Design review of the part built by this model. Coordinates are the model's own, in mm. Face numbers are marked on the shaded views. Coordinates: 2 decimals unless noted, no trailing zeros. Loops run counter-clockwise (first coordinate to the right, second up) from the corner with the lowest first, then second, coordinate; pieces in that order, holes last.
Q1. Add section B-B on x = 13. Give the boundary of the cut face in (y, z).
Q2. Add section D-D on x = -5. Give the boundary of the cut face in (y, z).
Q3. Add section C-C on z = 0. Give the boundary of the cut face in (x, y), and give its area (3 significant figures).
Q4. Wall thickness on probe 1 along Z at (x, y) = (0, -1.5); probe 2 along X at (y, z) = (-1.5, 22.5); probe 3 along Z at (x, y) = (3, -0.5): over which ranges is each line inside the solid? List them lowest first.
Q5. Draft analysis for pull direction X (two halves, no side actions). For the marked faces 1, 2 and 3, state which applies: released by +X, released by -X, zero draft, split by the parting line, or undercut.
Q6. Add section A-A on x = 0. Give the boundary of the cut face in (y, z).
Q7. For P1, Ø2, axis at x = -11.5, y = 1, coming from the +Z side; P2, Ø1, axis at x = -3.5, y = -1, coming from the -Z side; P3, Ø3.5, axis at x = -2.5, z = 23, coming from the -Y side; P4, Ø5, axis at x = 0, z = -21.5, coming from the +Y side, all flat-tipped, find the tip position at first contact; note any pin that passes through.
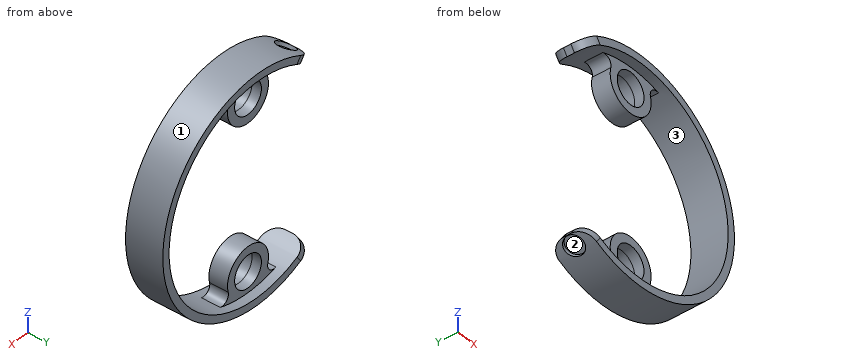
Autodesk Inventor part; units mm, degrees
ref_plane "YZ Plane" through (0, 0, 0) normal (1, 0, 0) x (0, 1, 0)
ref_plane "XZ Plane" through (0, 0, 0) normal (0, 1, 0) x (-1, 0, 0)
ref_plane "XY Plane" through (0, 0, 0) normal (0, 0, 1) x (1, 0, 0)
sketch "Skizze1" plane through (0, 0, 0) normal (0, 1, 0) x (-1, 0, 0)
  circle A0 centre (0, 0) radius 28
  circle A1 centre (0, 0) radius 30
  dimension "d0" = 56
  dimension "d1" = 60
extrude "Extrusion1" add sketch "Skizze1" along normal mid plane 10
sketch "Skizze2" plane through (0, 0, 0) normal (0, 1, 0) x (-1, 0, 0)
  circle A0 centre (0, 22.5) radius 4.25
  circle A1 centre (0, -22.5) radius 4.25
  line L0 (44.9262, 0) -> (-43.1306, 0) construction
  circle A2 centre (0, -22.5) radius 6.5
  circle A3 centre (0, 22.5) radius 6.5
  line L1 (0, 38.6377) -> (0, -60.2779) construction
  line L2 (3, 29.5) -> (-3, 29.5)
  line L3 (-3, 29.5) -> (-3, -29.5)
  line L4 (-3, -29.5) -> (3, -29.5)
  line L5 (3, -29.5) -> (3, 29.5)
  point P0 (0, 0)
  point P1 (-3, 28.2663)
  point P2 (3, 28.2663)
  point P3 (-3, -28.2663)
  point P4 (3, -28.2663)
  dimension "d4" = 45
  dimension "d5" = 8.5
  dimension "d6" = 8.5
  dimension "d7" = 13
  dimension "d8" = 13
  dimension "d9" = 6
  dimension "d21" = 59
extrude "Extrusion2" add sketch "Skizze2" along normal mid plane 5 contours A0 L5 A3 | A0 L3 A3 L5 | L5 A3 L3 A0 | A0 L3 A3 | A3 L3 L2 L5 | L5 A1 L3 A2 | A2 L5 A1 | L3 A1 A2 | L3 A1 L5 A2 | A2 L5 L4 L3
sketch "Skizze3" plane through (0, 0, 0) normal (0, 1, 0) x (-1, 0, 0)
  line L0 (-37.328, 53.3099) -> (47.5678, -67.9338) construction
  line L1 (48.5469, 69.3321) -> (-29.5635, -42.2211) construction
  line L2 (0, 56.0595) -> (0, -79.5026) construction
  circle A0 centre (0, 0) radius 30
  circle A1 centre (0, 0) radius 28
  line L3 (19.8236, 28.311) -> (13.732, 19.6114)
  line L4 (14.4871, -20.6897) -> (22.3283, -31.8882)
  point P0 (16.0601, -22.9363)
  point P1 (17.2073, -24.5746)
  point P2 (17.2073, 24.5746)
  point P3 (16.0601, 22.9363)
  dimension "d12" = 110
  dimension "d13" = 35
  dimension "d19" = 56
  dimension "d20" = 60
extrude "Extrusion3" cut sketch "Skizze3" along normal mid plane 10 contours A0 L4 A1 L3 picked at (29.0468, 2.3769)
sketch "Skizze4" plane through (0, 0, 0) normal (0, 1, 0) x (-1, 0, 0)
  line L0 (-8.0451, 13.9345) -> (38.1422, -66.0642) construction
  line L1 (17.2073, -24.5746) -> (16.0601, -22.9363) construction
  line L2 (0, 9.2259) -> (0, -51.7672) construction
  arc A0 (17.2073, 24.5746) -> (17.2073, -24.5746) centre (0, 0) ccw
  point P0 (16.6337, -23.7554)
  point P1 (15, -25.9808)
  point P2 (15, -25.9808)
  point P3 (19.2393, -22.9285)
  dimension "d16" = 30
ref_plane "Arbeitsebene3" through (-15.5, 0, -26.8468) normal (-0.4226, 0, -0.9063) x (0, -1, 0)
sketch "Skizze5" plane through (-15.5, 0, -26.8468) normal (-0.4226, 0, -0.9063) x (0, -1, 0)
  point P0 (0, -2.7018)
ref_plane "Arbeitsebene4" through (-15, 0, -25.9808) normal (-0.5, 0, -0.866) x (0, -1, 0)
sketch "Skizze6" plane through (-15, 0, -25.9808) normal (-0.5, 0, -0.866) x (0, -1, 0)
  circle A0 centre (0, 0) radius 2.5131
  point P0 (0, 0)
extrude "Extrusion5" cut sketch "Skizze6" against normal blind 1
mirror "Spiegeln2" about plane through (0, 0, 0) normal (0, 0, 1) of "Extrusion5"
fillet "Rundung1" radius 4 4 edges at (-16.6337, -5, -23.7554) (-16.6337, 5, -23.7554) (-16.6337, 5, 23.7554) (-16.6337, -5, 23.7554)
fillet "Rundung2" radius 2 4 edges at (3.8552, 0, -27.7333) (-3.8552, 0, -27.7333) (-3.8552, 0, 27.7333) (3.8552, 0, 27.7333)
ref_plane "Arbeitsebene5" through (0, 0, 0) normal (0, 0, 1) x (1, 0, 0)
properties part number "_3D-Druck"
Entries:
1. outline: (-5, -27.04) - (5, -27.04) - (5, -24.8) - (-5, -24.8) - close; (-5, 24.8) - (5, 24.8) - (5, 27.04) - (-5, 27.04) - close
2. outline: (-5, -29.58) - (5, -29.58) - (5, -27.55) - (2.5, -27.55) - (2.5, -18.35) - (-2.5, -18.35) - (-2.5, -27.55) - (-5, -27.55) - close; (-5, 27.55) - (-2.5, 27.55) - (-2.5, 18.35) - (2.5, 18.35) - (2.5, 27.55) - (5, 27.55) - (5, 29.58) - (-5, 29.58) - close
3. outline: (28, -5) - (30, -5) - (30, 5) - (28, 5) - close
3. area: 20.0 mm2
4. probe 1: z = -30 to -26.75, -18.25 to -16, 16 to 18.25, 26.75 to 30
4. probe 2: x = -6.5 to -4.25, 4.25 to 6.5, 16.67 to 19.84
4. probe 3: z = -29.85 to -25.51, -19.49 to -16.73, 16.73 to 19.49, 25.51 to 29.85
5. face 1: split by the parting line
5. face 2: undercut
5. face 3: undercut
6. outline: (-5, -30) - (5, -30) - (5, -28) - (2.5, -28) - (2.5, -26.75) - (-2.5, -26.75) - (-2.5, -28) - (-5, -28) - close; (-5, 28) - (-2.5, 28) - (-2.5, 26.75) - (2.5, 26.75) - (2.5, 28) - (5, 28) - (5, 30) - (-5, 30) - close; (-2.5, -18.25) - (2.5, -18.25) - (2.5, -16) - (-2.5, -16) - close; (-2.5, 16) - (2.5, 16) - (2.5, 18.25) - (-2.5, 18.25) - close
7. P1: stops at z = 28.1
7. P2: stops at z = -29.85
7. P3: stops at y = -2.5
7. P4: passes through
